Geometry check sheet. Reference: the model listing, model coordinates, mm. A direction names the side the tool comes from. Coordinates: 2 decimals unless noted, no trailing zeros. Loops run counter-clockwise (first coordinate to the right, second up) from the corner with the lowest first, then second, coordinate; pieces in that order, holes last.
Autodesk Inventor part; units mm, degrees
ref_plane "YZ Plane" through (0, 0, 0) normal (1, 0, 0) x (0, 1, 0)
ref_plane "XZ Plane" through (0, 0, 0) normal (0, 1, 0) x (-1, 0, 0)
ref_plane "XY Plane" through (0, 0, 0) normal (0, 0, 1) x (1, 0, 0)
sketch "Sketch1" plane through (0, 0, 0) normal (0, 0, 1) x (1, 0, 0)
  line L0 (0, 0) -> (0, 22.225)
  line L1 (0, 22.225) -> (-3.175, 22.225)
  circle A0 centre (-3.175, 22.225) radius 2.1082
  circle A1 centre (0, 0) radius 2.1082
  line L2 (0, 0) -> (7.62, 0)
  line L3 (7.62, 0) -> (7.62, -7.62)
  line L4 (7.62, -7.62) -> (0, -7.62)
  line L5 (0, -7.62) -> (0, 0)
  line L6 (-3.175, 22.225) -> (-13.335, 22.225)
  line L7 (-13.335, 22.225) -> (-13.335, 29.845)
  line L8 (-13.335, 29.845) -> (-3.175, 29.845)
  line L9 (-3.175, 29.845) -> (-3.175, 22.225)
  line L10 (-13.335, 29.845) -> (7.62, 29.845)
  line L11 (7.62, 29.845) -> (7.62, -7.62)
  line L12 (7.62, -7.62) -> (-13.335, -7.62)
  line L13 (-13.335, -7.62) -> (-13.335, 29.845)
  line L14 (-13.335, 29.845) -> (-20.955, 29.845)
  line L15 (-20.955, 29.845) -> (-20.955, -7.62)
  line L16 (-20.955, -7.62) -> (-13.335, -7.62)
  line L17 (-13.335, -7.62) -> (-13.335, 29.845)
  point P0 (-3.175, 29.845)
  point P1 (-13.335, -7.62)
  dimension "d0" = 22.225
  dimension "d1" = 3.175
  dimension "d2" = 4.2164
  dimension "d3" = 4.2164
  dimension "d4" = 7.62
  dimension "d5" = 7.62
  dimension "d6" = 10.16
  dimension "d7" = 7.62
  dimension "d8" = 7.62
extrude "Extrusion1" add sketch "Sketch1" along normal blind 12.7 contours A1 L5 L12 L13 L6 A0 L1 L0 | L0 L1 A0 L9 L10 L11 L2 A1 | L2 L3 L4 L5 A1 | L16 L15 L14 L7 L13 | A0 L6 L7 L8 L9
sketch "Sketch2" plane through (0, 0, 12.7) normal (0, 0, 1) x (1, 0, 0)
  line L0 (-20.955, 29.845) -> (-20.955, -7.62)
  line L1 (-20.955, 29.845) -> (-10.795, 29.845)
  line L2 (-10.795, 29.845) -> (-10.795, 4.445)
  line L3 (-10.795, 4.445) -> (-20.955, 4.445)
  line L4 (-20.955, 4.445) -> (-20.955, 29.845)
  point P0 (0, 0)
  point P1 (-20.955, 4.445)
  dimension "d11" = 10.16
  dimension "d12" = 25.4
extrude "Extrusion2" cut sketch "Sketch2" against normal blind 31.75
fillet "Fillet1" radius 3.175 1 edges at (-10.795, 4.445, 6.35)
sketch "Sketch3" plane through (-20.955, -7.62, 0) normal (-1, 0, 0) x (0, 0, 1)
  point P0 (0, 7.62)
sketch "Sketch4" plane through (-20.955, -7.62, 0) normal (-1, 0, 0) x (0, 0, 1)
  line L0 (0, 12.065) -> (0, 0)
  line L1 (0, 12.065) -> (12.7, 12.065)
  line L2 (0, 0) -> (12.7, 0)
  line L3 (12.7, 0) -> (12.7, 12.065)
  line L4 (12.7, 12.065) -> (0, 12.065)
  line L5 (0, 12.065) -> (0, 0)
  point P0 (0, 7.62)
extrude "Extrusion3" add sketch "Sketch4" along normal blind 5.08
sketch "Sketch5" plane through (-13.97, 4.445, 12.7) normal (0, 1, 0) x (1, 0, 0)
  line L0 (-12.065, 0) -> (-12.065, 12.7)
  line L1 (0, 0) -> (-12.065, 0)
  line L2 (-12.065, 12.7) -> (0, 0)
  circle A0 centre (-6.0325, 6.35) radius 2.1082
  point P0 (13.97, 12.7)
  dimension "d18" = 4.2164
extrude "Extrusion4" cut sketch "Sketch5" against normal blind 20.32 contours A0 L2 | L2 A0
fillet "Fillet2" radius 1.5875 12 edges at (-11.7249, 5.3749, 12.7) (-10.795, 18.7325, 12.7) (-20.0025, 4.445, 12.7) (-10.795, 29.845, 6.35) (-1.5875, 29.845, 12.7) (7.62, 29.845, 6.35) (7.62, 11.1125, 12.7) (-9.2075, -7.62, 12.7) (-26.035, -1.5875, 12.7) (-26.035, -7.62, 6.35) (-26.035, 4.445, 6.35) (7.62, -7.62, 6.35)
properties part number "wing arm mount (left)"
(1) Draft check along Z on faces 1 (the cylindrical face through (7.14, 11.35, 12.25)), 2 (the flat face through (-9, -7.62, 5)), 3 (the cylindrical face through (-17.99, -1.5, 5.72)). Enter one of: +Z half, -Z half, draft (parallel to the pull), parting line (faces both ways), or undercut.
Findings:
face 1: +Z half
face 2: draft
face 3: undercut
(2) Sectioned sample at C-C on x = -20. Record the cut outline in (y, z) (1 decimal), and give its area (3 significant figures).
Findings:
outline: (-7.6, 0) - (4.4, 0) - (4.4, 4.2) - (-7.6, 4.2) - close; (-7.6, 8.5) - (4.4, 8.5) - (4.4, 11.1) arc R1.6 ccw to (2.9, 12.7) - (-6, 12.7) arc R1.6 ccw to (-7.6, 11.1) - close
area: 101 mm2
(3) Sectioned sample at A-A on y = 0. State how many separate pieces and enclosed holes the cut face has, and give its area (3 significant figures).
Findings:
separate pieces: 2
enclosed holes: 1
area: 359 mm2
(4) Gauge pin test, flat ends, axial feed: pin 1 Ø3 at (x, z) = (-17.5, 8) entering from +Y (3 decimals); pin 2 Ø2.5 at (x, y) = (0, 0) entering from +Z. Record the tip position at first contact, or that the pin passes through.
Findings:
pin 1: stops at y = 4.445
pin 2: passes through
(5) Access from +Z, -Z, +X, -X, +Y, -Y to the whole of each face (thin tool, end or side, straight path). Record for faces 4 (the flat face through (-18, 4.445, 5)), 5 (the cylindrical face through (-4.73, 20.8, 6.26)), 6 (the cylindrical face through (-19.135, 3.992, 12.223)).
Findings:
face 4: +Z, -Z, -X, +Y
face 5: +Z, -Z
face 6: +Z, -X, +Y
(6) Scan lines: L1, parallel to X at y = -3.25, z = 6.35 (3 decimals); L2, parallel to X at y = 0.5, z = 6.35 (3 decimals); L3, parallel to Y at x = -3, z = 9 (3 decimals). Record each from-to range of solid material in increasing order.
Findings:
L1: x = -26.035 to -22.111, -17.894 to 7.62
L2: x = -26.035 to -22.111, -17.894 to -2.048, 2.048 to 7.62
L3: y = -7.62 to 20.124, 24.326 to 29.845
